The listing builds one solid part. Answer for the finished solid, in the listing's coordinates (mm). Coordinates: 2 decimals unless noted, no trailing zeros. Order: outer loops, then holes, each group sorted by start corner. A loop starts at its lowest first (then second) coordinate and runs counter-clockwise, first axis right, second up.
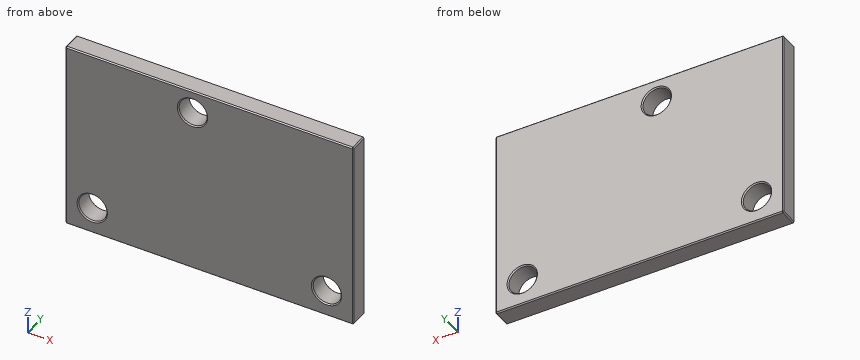
from build123d import *

# Parameters (mm, degrees)
SKETCH1_W           = 750
SKETCH1_H           = 500
BOSS_EXTRUDE1_DEPTH = 50
CUT_EXTRUDE1_REACH  = 455.459
SKETCH2_R           = 36.5
CHAMFER1_SIZE       = 3
CHAMFER2_SIZE       = 3


with BuildPart() as part:
    # Sketch1 → Boss-Extrude1 (new body)
    with BuildSketch(Plane(origin=(0, 0, 0), x_dir=(1, 0, 0), z_dir=(0, 1, 0))):
        Rectangle(SKETCH1_W, SKETCH1_H)
    extrude(amount=-BOSS_EXTRUDE1_DEPTH)

    # Sketch2 → Cut-Extrude1 (cut, up to next)
    with BuildSketch(Plane(origin=(0, 0, 0), x_dir=(1, 0, 0), z_dir=(0, 1, 0)), mode=Mode.PRIVATE) as cut_extrude1_sk1:
        with Locations(Location((-305, 180, 0), (0, 0, 270))):
            Circle(SKETCH2_R)
    cut_extrude1_tool1 = extrude(cut_extrude1_sk1.sketch, amount=-CUT_EXTRUDE1_REACH, mode=Mode.PRIVATE) & part.part
    # Sketch2 → Cut-Extrude1 (cut, up to next)
    with BuildSketch(Plane(origin=(0, 0, 0), x_dir=(1, 0, 0), z_dir=(0, 1, 0)), mode=Mode.PRIVATE) as cut_extrude1_sk2:
        with Locations(Location((305, 180, 0), (0, 0, 270))):
            Circle(SKETCH2_R)
    cut_extrude1_tool2 = extrude(cut_extrude1_sk2.sketch, amount=-CUT_EXTRUDE1_REACH, mode=Mode.PRIVATE) & part.part
    # Sketch2 → Cut-Extrude1 (cut, up to next)
    with BuildSketch(Plane(origin=(0, 0, 0), x_dir=(1, 0, 0), z_dir=(0, 1, 0)), mode=Mode.PRIVATE) as cut_extrude1_sk3:
        with Locations(Location((-44, -190, 0), (0, 0, 270))):
            Circle(SKETCH2_R)
    cut_extrude1_tool3 = extrude(cut_extrude1_sk3.sketch, amount=-CUT_EXTRUDE1_REACH, mode=Mode.PRIVATE) & part.part
    add(cut_extrude1_tool1.solids().sort_by_distance((-305, 0, -180))[0], mode=Mode.SUBTRACT)
    add(cut_extrude1_tool2.solids().sort_by_distance((305, 0, -180))[0], mode=Mode.SUBTRACT)
    add(cut_extrude1_tool3.solids().sort_by_distance((-44, 0, 190))[0], mode=Mode.SUBTRACT)

    # Chamfer1
    chamfer1_edges = [part.edges().sort_by_distance(p)[0] for p in [
        (-305, -50, -216.5),
        (-305, 0, -216.5),
        (305, -50, -216.5),
        (305, 0, -216.5),
        (-44, -50, 153.5),
        (-44, 0, 153.5),
    ]]
    chamfer(chamfer1_edges, length=CHAMFER1_SIZE)

    # Chamfer2
    chamfer2_edges = [part.edges().sort_by_distance(p)[0] for p in [
        (-375, -50, 0),
        (0, -50, 250),
        (375, -50, 0),
        (0, 0, 250),
        (-375, 0, 0),
        (0, 0, -250),
        (375, 0, 0),
        (375, -25, 250),
        (-375, -25, 250),
        (-375, -25, -250),
        (375, -25, -250),
        (0, -50, -250),
    ]]
    chamfer(chamfer2_edges, length=CHAMFER2_SIZE)


solid = part.part
(1) Find the intervals of material crossed by probe 1 along X at (y, z) = (-12.5, -180); probe 2 along X at (y, z) = (-13, 190); probe 3 along Z at (x, y) = (-303.5, -25), in increasing order.
(2) Find section C-C on z = -180. Determine the outline of the cut face in (x, y), then the cut area to 3 significant figures.
(3) Find section A-A on y = -36. Determine the outline of the cut face in (x, z).
(4) Find section B-B on z = 190. Determine the outline of the cut face in (x, y).
(5) Find section D-D on x = 305. Determine the outline of the cut face in (y, z), then the cut area to 3 significant figures.
Resolved:
1. probe 1: x = -375 to -341.5, -268.5 to 268.5, 341.5 to 375
1. probe 2: x = -375 to -80.5, -7.5 to 375
1. probe 3: z = -250 to -216.47, -143.53 to 250
2. outline: (-375, -47) - (-372, -50) - (-344.5, -50) - (-341.5, -47) - (-341.5, -3) - (-344.5, 0) - (-372, 0) - (-375, -3) - close; (-268.5, -47) - (-265.5, -50) - (265.5, -50) - (268.5, -47) - (268.5, -3) - (265.5, 0) - (-265.5, 0) - (-268.5, -3) - close; (341.5, -47) - (344.5, -50) - (372, -50) - (375, -47) - (375, -3) - (372, 0) - (344.5, 0) - (341.5, -3) - close
2. area: 30,100 mm2
3. outline: (-375, -247) - (-372, -250) - (372, -250) - (375, -247) - (375, 247) - (372, 250) - (-372, 250) - (-375, 247) - close; hole circle Ø73 at (-305, -180); hole circle Ø73 at (-44, 190); hole circle Ø73 at (305, -180)
4. outline: (-375, -47) - (-372, -50) - (-83.5, -50) - (-80.5, -47) - (-80.5, -3) - (-83.5, 0) - (-372, 0) - (-375, -3) - close; (-7.5, -47) - (-4.5, -50) - (372, -50) - (375, -47) - (375, -3) - (372, 0) - (-4.5, 0) - (-7.5, -3) - close
5. outline: (-50, -247) - (-47, -250) - (-3, -250) - (0, -247) - (0, -219.5) - (-3, -216.5) - (-47, -216.5) - (-50, -219.5) - close; (-50, -140.5) - (-47, -143.5) - (-3, -143.5) - (0, -140.5) - (0, 247) - (-3, 250) - (-47, 250) - (-50, 247) - close
5. area: 21,300 mm2
